Verification items for the finished model (mm, model axes). A direction names the side the tool comes from. Give positions to 0.01 mm unless a question says otherwise; leave off trailing zeros. Loops run counter-clockwise (first coordinate to the right, second up) from the corner with the lowest first, then second, coordinate; pieces in that order, holes last. Notation, with made-up numbers: (78, 70) - (121, 70) arc R15 ccw to (121, 79) - close; hole circle Ø7 at (44.5, -8.75). An arc over 180 degrees is marked (long way). Answer in a Markdown table with one row per item.
```python
from build123d import *

# Parameters (mm, degrees)
SKETCH1_W           = 5.08
SKETCH1_H           = 5.08
BOSS_EXTRUDE1_DEPTH = 5.715
SKETCH2_W           = 86.36
SKETCH2_H           = 86.36
BOSS_EXTRUDE2_DEPTH = 5.08
FILLET1_R           = 5.08
SKETCH3_W           = 76.2
SKETCH3_H           = 76.2
BOSS_EXTRUDE3_DEPTH = 3


with BuildPart() as part:
    # Sketch1 → Boss-Extrude1 (new body)
    with BuildSketch(Plane(origin=(0, 0, 0), x_dir=(1, 0, 0), z_dir=(0, 1, 0))):
        Polygon((-5.08, 0), (0, 0), (0, 76.2), (76.2, 76.2), (76.2, 81.28), (-5.08, 81.28), align=None)
        Polygon((76.2, 0), (0, 0), (0, -5.08), (81.28, -5.08), (81.28, 76.2), (76.2, 76.2), align=None)
        with Locations((-2.54, -2.54)):
            Rectangle(SKETCH1_W, SKETCH1_H)
        with Locations((78.74, 78.74)):
            Rectangle(SKETCH1_W, SKETCH1_H)
    extrude(amount=-BOSS_EXTRUDE1_DEPTH)

    # Sketch2 → Boss-Extrude2 (add)
    with BuildSketch(Plane(origin=(0, -5.715, 0), x_dir=(-1, 0, 0), z_dir=(0, -1, 0))):
        with Locations((-38.1, 38.1)):
            Rectangle(SKETCH2_W, SKETCH2_H)
    extrude(amount=BOSS_EXTRUDE2_DEPTH)

    # Fillet1
    fillet1_edges = [part.edges().sort_by_distance(p)[0] for p in [
        (-5.08, -5.3975, 5.08),
        (-5.08, -5.3975, -81.28),
        (81.28, -5.3975, -81.28),
        (81.28, -5.3975, 5.08),
        (-5.08, -10.795, -38.1),
        (38.1, -10.795, -81.28),
        (81.28, -10.795, -38.1),
        (38.1, -10.795, 5.08),
    ]]
    fillet(fillet1_edges, radius=FILLET1_R)

    # Sketch3 → Boss-Extrude3 (add)
    with BuildSketch(Plane(origin=(0, -5.715, 0), x_dir=(1, 0, 0), z_dir=(0, 1, 0))):
        with Locations((38.1, 38.1)):
            Rectangle(SKETCH3_W, SKETCH3_H)
    extrude(amount=BOSS_EXTRUDE3_DEPTH)


solid = part.part
```
Q1. Sectioned sample at B-B (z = -13.5). Record the cut outline in (x, y) (3 decimals), and give its area (3 significant figures).
Completed:
| item | result |
|---|---|
| outline | (-5.08, -5.715) arc R5.08 ccw to (0, -10.795) - (76.2, -10.795) arc R5.08 ccw to (81.28, -5.715) - (81.28, 0) - (76.2, 0) - (76.2, -2.715) - (0, -2.715) - (0, 0) - (-5.08, 0) - close |
| area | 714 mm^2 |
Q2. Sectioned sample at D-D (y = -9). Record the cut outline in (x, z).
Completed:
| item | result |
|---|---|
| outline | (-3.87, -76.2) arc R3.87 ccw to (0, -80.07) - (76.2, -80.07) arc R3.87 ccw to (80.07, -76.2) - (80.07, 0) arc R3.87 ccw to (76.2, 3.87) - (0, 3.87) arc R3.87 ccw to (-3.87, 0) - close |
Q3. Draft check along Z on faces 3 (the face through (-3.552, -2.898, 3.631)), 4 (the face through (38, -2.715, -39)), 5 (the face through (81.28, -3, -38)). Enter one of: +Z half, -Z half, draft (parallel to the pull), parting line (faces both ways), or undercut.
Completed:
| item | result |
|---|---|
| face 3 | +Z half |
| face 4 | undercut |
| face 5 | draft |
Q4. Go/stop test with flat-tipped pins: P1, Ø8, axis at x = 21, z = -54.5, coming from the +Y side (3 decimals); P2, Ø1.5, axis at x = 56, y = -7.5, coming from the +Z side; P3, Ø1, axis at y = -6.5, z = -61.5, coming from the +X side. Record where each tip stops, or that it passes through.
Completed:
| item | result |
|---|---|
| P1 | y = -2.715 |
| P2 | z = 4.97 |
| P3 | x = 81.27 |
Q5. Tool access check on faces 1 (the face through (38, -1, -76.2)), 2 (the face through (79.831, -2.817, -79.752)). Record the directions out of +Z, -Z, +X, -X, +Y, -Y that give a thin tool (end or side, any length) a straight path to the whole face; none if there is none.
Completed:
| item | result |
|---|---|
| face 1 | +Y |
| face 2 | -Z, +X, +Y, -Y |
Q6. Thickness scan on line 1 (Z direction, x = 56, y = -0.5); line 2 (Y direction, x = 62, z = -13.5) (3 decimals); line 3 (X direction, y = -1.5, z = -74). Record the ranges inside material, lowest first.
Completed:
| item | result |
|---|---|
| line 1 | -81.28 to -76.2, 0 to 5.08 |
| line 2 | -10.795 to -2.715 |
| line 3 | -5.08 to 0, 76.2 to 81.28 |
Q7. Sectioned sample at A-A (y = -1.5). Record the cut outline in (x, z).
Completed:
| item | result |
|---|---|
| outline | (-5.08, -76.2) arc R5.08 ccw to (0, -81.28) - (76.2, -81.28) arc R5.08 ccw to (81.28, -76.2) - (81.28, 0) arc R5.08 ccw to (76.2, 5.08) - (0, 5.08) arc R5.08 ccw to (-5.08, 0) - close; hole (0, -76.2) - (76.2, -76.2) - (76.2, 0) - (0, 0) - close |
Q8. Sectioned sample at C-C (x = 2). Record the cut outline in (y, z) (3 decimals), and give its area (3 significant figures).
Completed:
| item | result |
|---|---|
| outline | (-10.795, -76.2) arc R5.08 ccw to (-5.715, -81.28) - (0, -81.28) - (0, -76.2) - (-2.715, -76.2) - (-2.715, 0) - (0, 0) - (0, 5.08) - (-5.715, 5.08) arc R5.08 ccw to (-10.795, 0) - close |
| area | 714 mm^2 |
